```python
from build123d import *

# Parameters (mm, degrees)
SKETCH1_W           = 143
SKETCH1_H           = 101
BOSS_EXTRUDE1_DEPTH = 4
SKETCH2_W           = 155
SKETCH2_H           = 115
BOSS_EXTRUDE2_DEPTH = 4
FILLET1_R           = 5
FILLET2_R           = 1
SKETCH3_W           = 150
SKETCH3_H           = 110
BOSS_EXTRUDE3_DEPTH = 5


with BuildPart() as part:
    # Sketch1 → Boss-Extrude1 (new body)
    with BuildSketch(Plane(origin=(0, 0, 0), x_dir=(1, 0, 0), z_dir=(0, 1, 0))):
        Rectangle(SKETCH1_W, SKETCH1_H)
    extrude(amount=BOSS_EXTRUDE1_DEPTH)

    # Sketch2 → Boss-Extrude2 (add)
    with BuildSketch(Plane(origin=(0, 4, 0), x_dir=(1, 0, 0), z_dir=(0, 1, 0))):
        Rectangle(SKETCH2_W, SKETCH2_H)
    extrude(amount=BOSS_EXTRUDE2_DEPTH)

    # Fillet1
    fillet1_edges = [part.edges().sort_by_distance(p)[0] for p in [
        (71.5, 2, 50.5),
        (-71.5, 2, 50.5),
        (-71.5, 2, -50.5),
        (71.5, 2, -50.5),
    ]]
    fillet(fillet1_edges, radius=FILLET1_R)

    # Fillet2
    fillet2_edges = [part.edges().sort_by_distance(p)[0] for p in [
        (-77.5, 6, -57.5),
        (-77.5, 6, 57.5),
        (77.5, 6, 57.5),
        (77.5, 6, -57.5),
    ]]
    fillet(fillet2_edges, radius=FILLET2_R)

    # Sketch3 → Boss-Extrude3 (add)
    with BuildSketch(Plane(origin=(0, 4, 0), x_dir=(-1, 0, 0), z_dir=(0, -1, 0))):
        with BuildLine():
            Line((-76.5, -57.5), (76.5, -57.5))
            ThreePointArc((76.5, -57.5), (77.207106781, -57.207106781), (77.5, -56.5))
            Line((77.5, -56.5), (77.5, 56.5))
            ThreePointArc((77.5, 56.5), (77.207106781, 57.207106781), (76.5, 57.5))
            Line((76.5, 57.5), (-76.5, 57.5))
            ThreePointArc((-76.5, 57.5), (-77.207106781, 57.207106781), (-77.5, 56.5))
            Line((-77.5, 56.5), (-77.5, -56.5))
            ThreePointArc((-77.5, -56.5), (-77.207106781, -57.207106781), (-76.5, -57.5))
        make_face()
        Rectangle(SKETCH3_W, SKETCH3_H, mode=Mode.SUBTRACT)
    extrude(amount=BOSS_EXTRUDE3_DEPTH)


solid = part.part
```
Input: part model. Units: mm. Frame: model coordinates. A direction names the side the tool comes from. Give positions to 0.01 mm unless a question says otherwise; leave off trailing zeros. Order: outer loops, then holes, each group sorted by start corner. A loop starts at its lowest first (then second) coordinate and runs counter-clockwise, first axis right, second up. Notation, with made-up numbers: (-14, 88) - (9, 88) arc R19 cw to (9, 93) - close; hole circle Ø2 at (24.5, 50). An arc over 180 degrees is marked (long way). Use a Markdown table: item, result.
(1) Section query B-B (x = 45). Output: boundary loops of the cut face in (y, z), then the cut area to 3 significant figures.
Computed values:
| item | result |
|---|---|
| outline | (-1, -57.5) - (8, -57.5) - (8, 57.5) - (-1, 57.5) - (-1, 55) - (4, 55) - (4, 50.5) - (0, 50.5) - (0, -50.5) - (4, -50.5) - (4, -55) - (-1, -55) - close |
| area | 889 mm2 |
(2) Access query for faces 5 (the flat face through (1, 4, 57.5)), 6 (the cylindrical face through (-70, 2.03, 49.07)). Directions: +Z, -Z, +X, -X, +Y, -Y. A direction counts if a zero-diameter tool reaches every point of the face in a straight line with its end or side. Return the directions, or none.
Computed values:
| item | result |
|---|---|
| face 5 | +Z, +X, -X, +Y, -Y |
| face 6 | -Y |
(3) Section query C-C (z = 36.5). Output: boundary loops of the cut face in (x, y), then the cut area to 3 significant figures.
Computed values:
| item | result |
|---|---|
| outline | (-77.5, -1) - (-75, -1) - (-75, 4) - (-71.5, 4) - (-71.5, 0) - (71.5, 0) - (71.5, 4) - (75, 4) - (75, -1) - (77.5, -1) - (77.5, 8) - (-77.5, 8) - close |
| area | 1,220 mm2 |
(4) Draft query along X for faces 1 (the flat face through (0, -1, -56)), 2 (the flat face through (-75, 2, 1)), 3 (the flat face through (71.5, 2, 1)), 4 (the flat face through (77.5, 4, -1)). Return one class per face: released by +X, released by -X, zero draft, split by the parting line, or undercut.
Computed values:
| item | result |
|---|---|
| face 1 | zero draft |
| face 2 | undercut |
| face 3 | undercut |
| face 4 | released by +X |
(5) Line query: line 1 (X direction, y = 2.5, z = 40.5); line 2 (Z direction, x = 0.5, y = 0.75); line 3 (X direction, y = 1.75, z = 50). Output: solid intervals per line, ascending. Write a range as from..to.
Computed values:
| item | result |
|---|---|
| line 1 | x = -77.5..-75, -71.5..71.5, 75..77.5 |
| line 2 | z = -57.5..-55, -50.5..50.5, 55..57.5 |
| line 3 | x = -77.5..-75, -68.68..68.68, 75..77.5 |
(6) Pin query (flat end, axial travel): pin 1 (12 mm diameter, centred on x = -5, z = -38.5, fed in from -Y). Return the tip coordinate at first contact, or that it passes through.
Computed values:
| item | result |
|---|---|
| pin 1 | stops at y = 0 |
(7) Section query A-A (y = 1.5). Output: boundary loops of the cut face in (x, z).
Computed values:
| item | result |
|---|---|
| outline | (-77.5, -56.5) arc R1 ccw to (-76.5, -57.5) - (76.5, -57.5) arc R1 ccw to (77.5, -56.5) - (77.5, 56.5) arc R1 ccw to (76.5, 57.5) - (-76.5, 57.5) arc R1 ccw to (-77.5, 56.5) - close; (-71.5, -45.5) arc R5 ccw to (-66.5, -50.5) - (66.5, -50.5) arc R5 ccw to (71.5, -45.5) - (71.5, 45.5) arc R5 ccw to (66.5, 50.5) - (-66.5, 50.5) arc R5 ccw to (-71.5, 45.5) - close; hole (-75, -55) - (75, -55) - (75, 55) - (-75, 55) - close |
